```python
from build123d import *

# Parameters (mm, degrees)
SKETCH1_R           = 18.5
SKETCH1_W           = 25.908
SKETCH1_H           = 25.908
BOSS_EXTRUDE1_DEPTH = 10
SKETCH2_R           = 26.5
SKETCH2_R_2         = 10
BOSS_EXTRUDE2_DEPTH = 5
SKETCH3_W           = 42.310591005
SKETCH3_H           = 3.35
FILLET1_R           = 10


with BuildPart() as part:
    # Sketch1 → Boss-Extrude1 (new, symmetric)
    with BuildSketch(Plane(origin=(0, 0, 0), x_dir=(1, 0, 0), z_dir=(0, 1, 0))):
        with BuildLine():
            Line((-18.754, -77.954), (18.754, -77.954))
            Line((18.754, -77.954), (18.754, -18.722646287))
            ThreePointArc((18.754, -18.722646287), (0, 26.5), (-18.754, -18.722646287))
            Line((-18.754, -18.722646287), (-18.754, -77.954))
        make_face()
        with Locations(Location((0, 0, 0), (0, 0, 270))):
            Circle(SKETCH1_R, mode=Mode.SUBTRACT)
        with Locations((0, -60)):
            Rectangle(SKETCH1_W, SKETCH1_H, mode=Mode.SUBTRACT)
    extrude(amount=BOSS_EXTRUDE1_DEPTH, both=True)

    # Sketch2 → Boss-Extrude2 (add)
    with BuildSketch(Plane(origin=(0, 10, 0), x_dir=(1, 0, 0), z_dir=(0, 1, 0))):
        Circle(SKETCH2_R)
        with Locations(Location((0, 0, 0), (0, 0, 270))):
            Circle(SKETCH2_R_2, mode=Mode.SUBTRACT)
    extrude(amount=-BOSS_EXTRUDE2_DEPTH)

    # Sketch3 → Cut-Revolve1 (revolve, cut)
    with BuildSketch(Plane(origin=(0, 0, 0), x_dir=(1, 0, 0), z_dir=(0, 1, 0))):
        with Locations((0.530790347, -58.325)):
            Rectangle(SKETCH3_W, SKETCH3_H)
    revolve(axis=Axis((-24.494150326, 0, 60), (1, 0, 0)), mode=Mode.SUBTRACT)

    # Fillet1
    fillet1_edges = [part.edges().sort_by_distance(p)[0] for p in [
        (18.754, 0, 18.722646287),
        (-18.754, 0, 18.722646287),
    ]]
    fillet(fillet1_edges, radius=FILLET1_R)


solid = part.part
```
The model under review builds one solid part; all positions refer to its coordinate system, in mm. A direction names the side the tool comes from. Round coordinates to 2 decimals unless told otherwise and drop trailing zeros. Loops run counter-clockwise (first coordinate to the right, second up) from the corner with the lowest first, then second, coordinate; pieces in that order, holes last. Notation, with made-up numbers: (-11, -25.5) - (20, -25.5) arc R34 cw to (20, 10.5) - close; hole circle Ø9 at (76.5, 8.5). An arc over 180 degrees is marked (long way). Write each question's results on one line, items separated by ' | '. Start each with the question number.
Q1. Take a section at D-D on x = 5. Give the boundary of the cut face in (y, z), plus the area to 3 significant figures.
Q2. Tool access review of faces 1 (the cylindrical face through (-15.813, 1.006, 56.805)), 2 (the cylindrical face through (-7.086, -2.605, 17.089)), 3 (the flat face through (-18.754, 0, 50)), 4 (the flat face through (18.754, 0, 51)), 5 (the flat face through (-12.954, 2, 57)): name each direction out of +Z, -Z, +X, -X, +Y, -Y from which nothing blocks a thin tool from reaching the whole face with its end or side.
Q3. Take a section at B-B on y = 0. Give the boundary of the cut face in (x, z).
Q4. Draft analysis for pull direction Z (two halves, no side actions). For faces 6 (the cylindrical face through (0.829, 0.14, -26.487)), 7 (the flat face through (12.954, 2, 57)), 8 (the flat face through (0, 0, 77.954)), state which applies: pulls with the +Z half, pulls with the -Z half, needs draft (parallel to the pull), parting line crosses it, or undercut.
Q5. Take a section at A-A on z = 60. Give the boundary of the cut face in (x, y).
Q6. Insertion check: P1, Ø12, axis at y = 1.5, z = 31, coming from the -X side; P2, Ø6, axis at x = 20.5, y = -3.5, coming from the -Z side; P3, Ø1.5, axis at y = -1, z = 10.5, coming from the -X side. Each pin has a flat end and moves straight along its axis. Give the tip position at first contact, or say it passes through.
Q7. Wall thickness on line 1 along Z through (x, y) = (10.5, -3.25); line 2 along Z through (x, y) = (9, 9.25); line 3 along Y through (x, z) = (17.15, 60): over which ranges is each line inside the solid? List them lowest first. Write a range as [from, to].
Q8. Take a section at C-C on z = 0. Give the boundary of the cut face in (x, y).
Data:
1) outline: (-10, -26.02) - (10, -26.02) - (10, -8.66) - (5, -8.66) - (5, -17.81) - (-10, -17.81) - close; (-10, 17.81) - (5, 17.81) - (5, 8.66) - (10, 8.66) - (10, 47.05) - (-10, 47.05) - close; (-10, 72.95) - (10, 72.95) - (10, 77.95) - (-10, 77.95) - close | area: 940 mm²
2) face 1: +X, -X | face 2: -Y | face 3: +Z, -X, +Y, -Y | face 4: +Z, +X, +Y, -Y | face 5: +Y, -Y
3) outline: (-20.88, 16.32) arc R26.5 ccw (long way) to (20.88, 16.32) arc R10 cw to (18.75, 22.48) - (18.75, 56.65) - (12.95, 56.65) - (12.95, 47.05) - (-12.95, 47.05) - (-12.95, 56.65) - (-18.75, 56.65) - (-18.75, 22.48) arc R10 cw to start; (-18.75, 63.35) - (-12.95, 63.35) - (-12.95, 72.95) - (12.95, 72.95) - (12.95, 63.35) - (18.75, 63.35) - (18.75, 77.95) - (-18.75, 77.95) - close; hole circle Ø37 at (0, 0)
4) face 6: parting line crosses it | face 7: undercut | face 8: pulls with the +Z half
5) outline: (-18.75, -10) - (-12.95, -10) - (-12.95, -3.35) - (-18.75, -3.35) - close; (-18.75, 3.35) - (-12.95, 3.35) - (-12.95, 10) - (-18.75, 10) - close; (12.95, -10) - (18.75, -10) - (18.75, -3.35) - (12.95, -3.35) - close; (12.95, 3.35) - (18.75, 3.35) - (18.75, 10) - (12.95, 10) - close
6) P1: stops at x = -18.75 | P2: stops at z = -19.9 | P3: stops at x = -24.64
7) line 1: z = [-24.33, -15.23], [15.23, 47.05], [72.95, 77.95] | line 2: z = [-24.92, -4.36], [4.36, 47.05], [72.95, 77.95] | line 3: y = [-10, -3.35], [3.35, 10]
8) outline: (-26.5, -10) - (-18.5, -10) - (-18.5, 5) - (-10, 5) - (-10, 10) - (-26.5, 10) - close; (10, 5) - (18.5, 5) - (18.5, -10) - (26.5, -10) - (26.5, 10) - (10, 10) - close
